Verification items for the finished model (mm, model axes). Face numbers are marked on the shaded views. Coordinates: 2 decimals unless noted, no trailing zeros. Write each loop counter-clockwise with the first axis right and the second up, starting at its lowest first coordinate (ties: lowest second). Pieces come first, ordered by that corner, then holes.
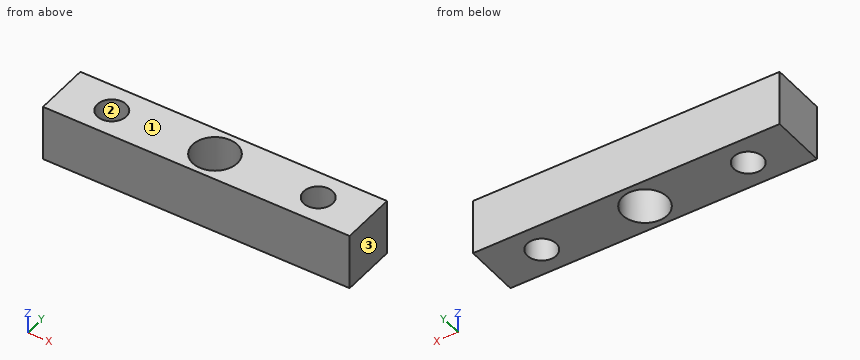
```python
from build123d import *

# Parameters (mm, degrees)
SKETCH_1_W          = 55
SKETCH_1_H          = 10
EXTRUDE_1_DEPTH     = 10
SKETCH_2_R          = 2.605
CUT_EXTRUDE_1_DEPTH = 10
SKETCH_3_R          = 4
CUT_EXTRUDE_2_DEPTH = 10


with BuildPart() as part:
    # 草图1 → 凸台-拉伸1 (new body)
    with BuildSketch(Plane.XY):
        Rectangle(SKETCH_1_W, SKETCH_1_H)
    extrude(amount=EXTRUDE_1_DEPTH)

    # 草图2 → 切除-拉伸1 (cut)
    with BuildSketch(Plane.XY.offset(10)):
        with Locations((18.515, 0)):
            Circle(SKETCH_2_R)
        with Locations((-18.515, 0)):
            Circle(SKETCH_2_R)
    extrude(amount=-CUT_EXTRUDE_1_DEPTH, mode=Mode.SUBTRACT)

    # 草图3 → 切除-拉伸2 (cut)
    with BuildSketch(Plane.XY.offset(10)):
        Circle(SKETCH_3_R)
    extrude(amount=-CUT_EXTRUDE_2_DEPTH, mode=Mode.SUBTRACT)


solid = part.part
```
1. Sectioned sample at C-C, the plane x = 0. Record the boundary of the cut face in (y, z).
2. Sectioned sample at B-B, the plane z = 9. Record the boundary of the cut face in (x, y) (3 decimals), and give its area (3 significant figures).
3. Material ranges on L1, parallel to X at y = 0.25, z = 7; L2, parallel to X at y = -0.75, z = 4; L3, parallel to Y at x = 0, z = 5.25, recorded low to high.
4. Sectioned sample at D-D, the plane x = -19. Record the boundary of the cut face in (y, z).
5. Sectioned sample at A-A, the plane y = 0. Record the boundary of the cut face in (x, z).
6. Gauge pin test, flat end, axial feed: P1, Ø4, axis at x = -18.515, y = 0, coming from the +Z side. Record the tip position at first contact, or that the pin passes through.
7. Draft check along X on the marked faces 1, 2 and 3. Enter one of: pulls with the +X half, pulls with the -X half, needs draft (parallel to the pull), parting line crosses it, or undercut.
Outcome:
1. outline: (-5, 0) - (-4, 0) - (-4, 10) - (-5, 10) - close; (4, 0) - (5, 0) - (5, 10) - (4, 10) - close
2. outline: (-27.5, -5) - (27.5, -5) - (27.5, 5) - (-27.5, 5) - close; hole circle Ø5.21 at (-18.515, 0); hole circle Ø8 at (0, 0); hole circle Ø5.21 at (18.515, 0)
2. area: 457 mm2
3. L1: x = -27.5 to -21.11, -15.92 to -3.99, 3.99 to 15.92, 21.11 to 27.5
3. L2: x = -27.5 to -21.01, -16.02 to -3.93, 3.93 to 16.02, 21.01 to 27.5
3. L3: y = -5 to -4, 4 to 5
4. outline: (-5, 0) - (-2.56, 0) - (-2.56, 10) - (-5, 10) - close; (2.56, 0) - (5, 0) - (5, 10) - (2.56, 10) - close
5. outline: (-27.5, 0) - (-21.12, 0) - (-21.12, 10) - (-27.5, 10) - close; (-15.91, 0) - (-4, 0) - (-4, 10) - (-15.91, 10) - close; (4, 0) - (15.91, 0) - (15.91, 10) - (4, 10) - close; (21.12, 0) - (27.5, 0) - (27.5, 10) - (21.12, 10) - close
6. P1: passes through
7. face 1: needs draft
7. face 2: undercut
7. face 3: pulls with the +X half
